Build history of the part. All positions in model axes, mm. A direction names the side the tool comes from. Round coordinates to 2 decimals unless told otherwise and drop trailing zeros. Loops run counter-clockwise (first coordinate to the right, second up) from the corner with the lowest first, then second, coordinate; pieces in that order, holes last. Notation, with made-up numbers: (-1.75, -35.5) - (38.25, -35.5) arc R24 cw to (38.25, -17.5) - close; hole circle Ø1 at (9.5, -4.75). An arc over 180 degrees is marked (long way). Put each result on its own line as item: value. Start each with the question number.
from build123d import *

# Parameters (mm, degrees)
SKETCH1_R                                            = 75
BOSS_EXTRUDE1_DEPTH                                  = 3
SKETCH2_R                                            = 10
SKETCH2_R_2                                          = 5.05
BOSS_EXTRUDE2_DEPTH                                  = 22
FILLET1_R                                            = 3
CUT_EXTRUDE1_DEPTH                                   = 76
CSK_FOR_M3_HEX_SOCKET_COUNTERSUNK_HEAD_S_D           = 3.6
CSK_FOR_M3_HEX_SOCKET_COUNTERSUNK_HEAD_S_CSINK_D     = 6.94
CSK_FOR_M3_HEX_SOCKET_COUNTERSUNK_HEAD_S_CSINK_ANGLE = 90


with BuildPart() as part:
    # Sketch1 → Boss-Extrude1 (new body)
    with BuildSketch(Plane(origin=(0, 0, 0), x_dir=(1, 0, 0), z_dir=(0, 1, 0))):
        Circle(SKETCH1_R)
    extrude(amount=BOSS_EXTRUDE1_DEPTH)

    # Sketch2 → Boss-Extrude2 (add)
    with BuildSketch(Plane(origin=(0, 3, 0), x_dir=(1, 0, 0), z_dir=(0, 1, 0))):
        Circle(SKETCH2_R)
        Circle(SKETCH2_R_2, mode=Mode.SUBTRACT)
    extrude(amount=BOSS_EXTRUDE2_DEPTH)

    # Fillet1
    fillet1_edges = [part.edges().sort_by_distance(p)[0] for p in [
        (-10, 3, 0),
    ]]
    fillet(fillet1_edges, radius=FILLET1_R)

    # Sketch3 → Cut-Extrude1 (cut, through all)
    with BuildSketch(Plane.XY):
        with BuildLine():
            Line((1.5, 25), (1.5, 6.5))
            ThreePointArc((1.5, 6.5), (0, 5), (-1.5, 6.5))
            Line((-1.5, 6.5), (-1.5, 25))
            ThreePointArc((-1.5, 25), (0, 26.5), (1.5, 25))
        make_face()
    extrude(amount=CUT_EXTRUDE1_DEPTH, mode=Mode.SUBTRACT)

    # CSK for M3 Hex Socket Countersunk Head Screw1 (through all)
    with Locations(Plane(origin=(0, 0, 0), x_dir=(-1, 0, 0), z_dir=(0, -1, 0))):
        with Locations((0, 0)):
            CounterSinkHole(CSK_FOR_M3_HEX_SOCKET_COUNTERSUNK_HEAD_S_D / 2, CSK_FOR_M3_HEX_SOCKET_COUNTERSUNK_HEAD_S_CSINK_D / 2, counter_sink_angle=CSK_FOR_M3_HEX_SOCKET_COUNTERSUNK_HEAD_S_CSINK_ANGLE)


solid = part.part
1) Slice it at B-B, the plane y = 21.25. Write the cut outline in (x, z), and give its area (3 significant figures).
2) Pull direction Z, two halves, no side cores. Call faces 4 (the face through (0, 15, -10)), 5 (the face through (1.5, 16, 7)), 6 (the face through (2.71, 13.85, -4.26)): pulls with the +Z half, pulls with the -Z half, needs draft (parallel to the pull), parting line crosses it, or undercut.
3) Which spindle directions (+Z, -Z, +X, -X, +Y, -Y) get a long thin tool onto all of the face, cutting with end or side? Do faces 1 (the face through (2, 3, 0)), 2 (the face through (1.717, 2.344, -0.541)), 3 (the face through (-1.5, 16, 7)). Say none if no direction does.
4) Drill centre lines: line 1 (Z direction, x = 0, y = 2.2); line 2 (Z direction, x = 0, y = 19.5); line 3 (Y direction, x = 9, z = 7). Where is each one in solid material? Low to high. Write a range as [from, to].
5) Slice it at A-A, the plane z = 0. Write the cut outline in (x, y).
6) Drop flat-ended pins along their axis: pin 1 Ø5.5 at (y, z) = (20, 7.5) entering from -X; pin 2 Ø4 at (y, z) = (18, 7) entering from +X; pin 3 Ø3 at (x, z) = (0, 0) entering from -Y; pin 4 Ø8 at (y, z) = (4, -11.5) entering from -X. Give the stop position or say it passes through.
7) Slice it at C-C, the plane x = 15.5. Write the cut outline in (y, z).
Taken from the geometry:
1. outline: (-1.5, 4.82) - (-1.5, 9.89) arc R10 ccw (long way) to (1.5, 9.89) - (1.5, 4.82) arc R5.05 cw (long way) to start
1. area: 219 mm2
2. face 4: parting line crosses it
2. face 5: needs draft
2. face 6: undercut
3. face 1: +Y
3. face 2: +Y, -Y
3. face 3: +Z, +Y
4. line 1: z = [-75, -1.8], [1.8, 75]
4. line 2: z = [-10, -5.05]
4. line 3: y = [0, 3.46]
5. outline: (-75, 0) - (-3.47, 0) - (-1.8, 1.67) - (-1.8, 3) - (-5.05, 3) - (-5.05, 25) - (-10, 25) - (-10, 6) arc R3 cw to (-13, 3) - (-75, 3) - close; (1.8, 1.67) - (3.47, 0) - (75, 0) - (75, 3) - (13, 3) arc R3 cw to (10, 6) - (10, 25) - (5.05, 25) - (5.05, 3) - (1.8, 3) - close
6. pin 1: stops at x = -8.8
6. pin 2: stops at x = 8.66
6. pin 3: passes through
6. pin 4: stops at x = -74.61
7. outline: (0, -73.38) - (3, -73.38) - (3, 73.38) - (0, 73.38) - close
